```python
from build123d import *

# Parameters (mm, degrees)
SKETCH_1_W          = 26
SKETCH_1_H          = 17.5
SKETCH_1_R          = 1.385
SKETCH_1_R_2        = 1.35
EXTRUDE_1_DEPTH     = 3
SKETCH_2_W          = 26
SKETCH_2_H          = 4
EXTRUDE_2_DEPTH     = 20
SKETCH_3_R          = 5
CUT_EXTRUDE_1_DEPTH = 20
EXTRUDE_3_DEPTH     = 3
EXTRUDE_4_DEPTH     = 3
EXTRUDE_5_DEPTH     = 3
EXTRUDE_6_DEPTH     = 3
FILLET_1_R          = 3


with BuildPart() as part:
    # Sketch 1 → Extrude 1 (new body)
    with BuildSketch(Plane(origin=(0, 0, 0), x_dir=(1, 0, 0), z_dir=(0, 1, 0))):
        Rectangle(SKETCH_1_W, SKETCH_1_H)
        with Locations(Location((-6, 2, 0), (0, 0, 270))):
            Circle(SKETCH_1_R, mode=Mode.SUBTRACT)
        with Locations(Location((-6, -6, 0), (0, 0, 270))):
            Circle(SKETCH_1_R_2, mode=Mode.SUBTRACT)
        with Locations(Location((6, 2, 0), (0, 0, 270))):
            Circle(SKETCH_1_R_2, mode=Mode.SUBTRACT)
        with Locations(Location((6, -6, 0), (0, 0, 270))):
            Circle(SKETCH_1_R_2, mode=Mode.SUBTRACT)
    extrude(amount=EXTRUDE_1_DEPTH)

    # Sketch 2 → Extrude 2 (add)
    with BuildSketch(Plane(origin=(0, 3, 0), x_dir=(1, 0, 0), z_dir=(0, 1, 0))):
        with Locations((0, 6.75)):
            Rectangle(SKETCH_2_W, SKETCH_2_H)
    extrude(amount=EXTRUDE_2_DEPTH)

    # Sketch 3 → Cut-Extrude 1 (cut)
    with BuildSketch(Plane.XY.offset(-4.75)):
        with Locations((0, 15)):
            Circle(SKETCH_3_R)
    extrude(amount=-CUT_EXTRUDE_1_DEPTH, mode=Mode.SUBTRACT)

    # Sketch 4 → Extrude 3 (add)
    with BuildSketch(Plane.ZY.offset(13)):
        Polygon((-8.75, 23), (-8.75, 0), (8.75, 0), (8.75, 3), (-4.75, 23), align=None)
    extrude(amount=EXTRUDE_3_DEPTH)

    # Sketch 5 → Extrude 4 (add)
    with BuildSketch(Plane(origin=(13, 0, 0), x_dir=(0, 0, -1), z_dir=(1, 0, 0))):
        Polygon((8.75, 0), (-8.75, 0), (-8.75, 3), (4.75, 23), (8.75, 23), align=None)
    extrude(amount=EXTRUDE_4_DEPTH)

    # Sketch 6 → Extrude 5 (add)
    with BuildSketch(Plane.ZY.offset(16)):
        Polygon((-4.75, 23), (8.75, 23), (8.75, 3), align=None)
    extrude(amount=-EXTRUDE_5_DEPTH)

    # Sketch 8 → Extrude 6 (add)
    with BuildSketch(Plane(origin=(16, 0, 0), x_dir=(0, 0, -1), z_dir=(1, 0, 0))):
        Polygon((-8.75, 3), (-8.75, 23), (4.75, 23), align=None)
    extrude(amount=-EXTRUDE_6_DEPTH)

    # Fillet 1
    fillet_1_edges = [part.edges().sort_by_distance(p)[0] for p in [
        (-13, 13, -4.75),
        (13, 13, -4.75),
    ]]
    fillet(fillet_1_edges, radius=FILLET_1_R)


solid = part.part
```
Here's how the part is built. I have some questions about the finished solid (model axes, mm). A direction names the side the tool comes from. Round coordinates to 2 decimals unless told otherwise and drop trailing zeros. Order: outer loops, then holes, each group sorted by start corner. A loop starts at its lowest first (then second) coordinate and runs counter-clockwise, first axis right, second up. Notation, with made-up numbers: (-2, -23.5) -> (17, -23.5) arc R8 cw to (17, -15.5) -> close; hole circle Ø2 at (76, 69). An arc over 180 degrees is marked (long way). Use a Markdown table: item, result. Add a question column.
(1) For pin 1 Ø4.5 at (x, z) = (-6, -2) entering from -Y; pin 2 Ø6 at (x, y) = (-8, 19.5) entering from +Z; pin 3 Ø4.5 at (x, z) = (6, -2) entering from +Y; pin 4 Ø10 at (x, y) = (5, 15.5) entering from +Z, each with a flat end and sliding along its axis, tell me the tip position at first contact or that it passes through.
(2) Suppose I cut it at B-B, the plane y = 15. Please give me the cut outline in (x, z).
(3) I need wall thicknesses on line 1 along X through (y, z) = (1.7, 6); line 2 along X through (y, z) = (0.65, -2) (3 decimals); line 3 along X through (y, z) = (15, 8). Which ranges of each line are inside material? Lowest first, please.
(4) Suppose I cut it at D-D, the plane z = -6. Please give me the cut outline in (x, y).
(5) For faces 1 (the face through (0, 0, 0)), 2 (the face through (12.14, 13.14, -3.85)), which set-ups out of +Z, -Z, +X, -X, +Y, -Y let a thin tool reach every point of the face, with its end or its side?
(6) If we mould it in two halves opening along X, with no side actions, what happens to faces 3 (the face through (-16, 12, 0)), 4 (the face through (0, 2, 8.75)), 5 (the face through (-12.1, 13.14, -3.89))? For each: released by +X, released by -X, zero draft, split by the parting line, or undercut.
(7) Suppose I cut it at A-A, the plane x = 6. Please give me the cut outline in (y, z).
(8) Suppose I cut it at C-C, the plane z = 6. Please give me the cut outline in (x, y).
Verdict:
| question | item | result |
|---|---|---|
| 1 | pin 1 | y = 0 |
| 1 | pin 2 | z = -4.58 |
| 1 | pin 3 | y = 3 |
| 1 | pin 4 | z = -4.75 |
| 2 | outline | (-16, -8.75) -> (-5, -8.75) -> (-5, -4.75) -> (-10, -4.75) arc R3 cw to (-13, -1.75) -> (-13, 8.75) -> (-16, 8.75) -> close; (5, -8.75) -> (16, -8.75) -> (16, 8.75) -> (13, 8.75) -> (13, -1.75) arc R3 cw to (10, -4.75) -> (5, -4.75) -> close |
| 3 | line 1 | -16 to -7.35, -4.65 to 4.65, 7.35 to 16 |
| 3 | line 2 | -16 to -7.385, -4.615 to 4.65, 7.35 to 16 |
| 3 | line 3 | -16 to -13, 13 to 16 |
| 4 | outline | (-16, 0) -> (16, 0) -> (16, 23) -> (-16, 23) -> close; hole circle Ø10 at (0, 15) |
| 5 | face 1 | +Z, -Z, +X, -X, -Y |
| 5 | face 2 | +Z, +Y |
| 6 | face 3 | released by -X |
| 6 | face 4 | zero draft |
| 6 | face 5 | undercut |
| 7 | outline | (0, -8.75) -> (23, -8.75) -> (23, -4.75) -> (3, -4.75) -> (3, -3.35) -> (0, -3.35) -> close; (0, -0.65) -> (3, -0.65) -> (3, 4.65) -> (0, 4.65) -> close; (0, 7.35) -> (3, 7.35) -> (3, 8.75) -> (0, 8.75) -> close |
| 8 | outline | (-16, 0) -> (-7.35, 0) -> (-7.35, 3) -> (-13, 3) -> (-13, 23) -> (-16, 23) -> close; (-4.65, 0) -> (4.65, 0) -> (4.65, 3) -> (-4.65, 3) -> close; (7.35, 0) -> (16, 0) -> (16, 23) -> (13, 23) -> (13, 3) -> (7.35, 3) -> close |
